Job drawing, mm, ordinate dimensions from the low corner. One solid piece. A direction names the side the tool comes from. Round coordinates to 2 decimals unless told otherwise and drop trailing zeros. Loops run counter-clockwise (first coordinate to the right, second up) from the corner with the lowest first, then second, coordinate; pieces in that order, holes last.
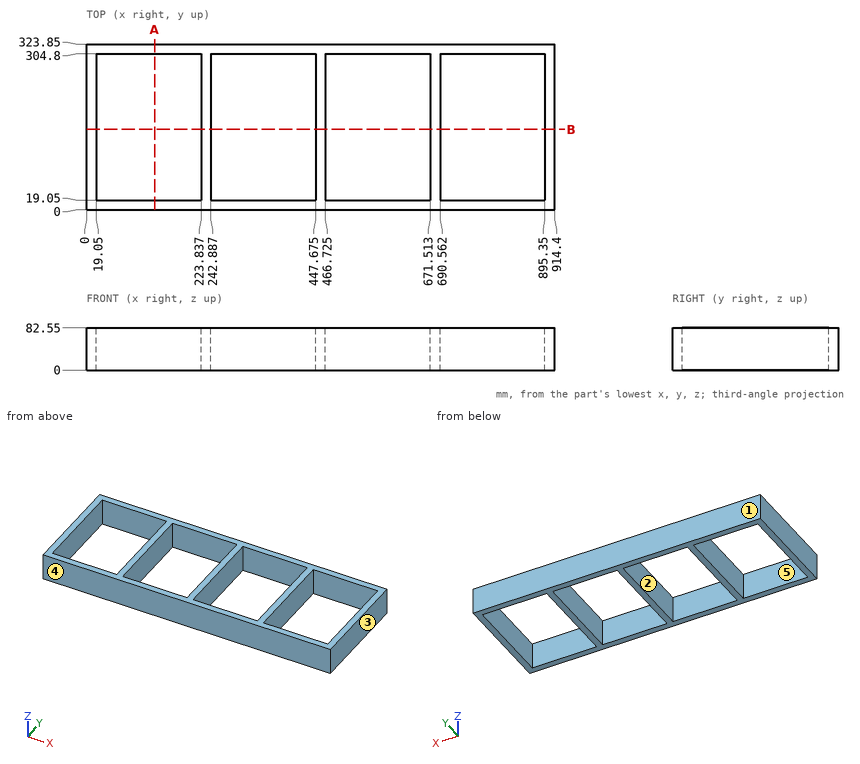
(1) Slice it at A-A on x = 133. List the corners of the cut face in (y, z).
Responses:
outline: (0, 0) - (19.05, 0) - (19.05, 82.55) - (0, 82.55) - close; (304.8, 0) - (323.85, 0) - (323.85, 82.55) - (304.8, 82.55) - close
(2) Pull direction X, two halves, no side cores. Call the marked faces 1, 2 and 3: +X half, -X half, draft (parallel to the pull), parting line (faces both ways), or undercut.
Responses:
face 1: draft
face 2: undercut
face 3: +X half
(3) Probe line 1 (Y direction, x = 115, z = 62). List the from-to ranges inside material, lowest first.
Responses:
line 1: y = 0 to 19.05, 304.8 to 323.85
(4) Which spindle directions (+Z, -Z, +X, -X, +Y, -Y) get a long thin tool onto all of the face, cutting with end or side? Do the marked faces 4 and 5. Say none if no direction does.
Responses:
face 4: +Z, -Z, +X, -X, -Y
face 5: +Z, -Z
(5) Slice it at B-B on y = 157. Count the separate pieces of the cut face and the enclosed holes in it, plus the area to 3 significant figures.
Responses:
separate pieces: 5
enclosed holes: 0
area: 7,860 mm2
